Here's the drawing with two shaded views (mm, measured from the low corner). I have some questions. A direction names the side the tool comes from. Coordinates: 2 decimals unless noted, no trailing zeros. Write each loop counter-clockwise with the first axis right and the second up, starting at its lowest first coordinate (ties: lowest second). Pieces come first, ordered by that corner, then holes. Notation, with made-up numbers: (7.5, -34.5) -> (26.5, -34.5) arc R14 ccw to (26.5, -16.5) -> close; hole circle Ø8 at (81, 62.25). An arc over 180 degrees is marked (long way). Answer in a Markdown table with one row per item. Add a question column.
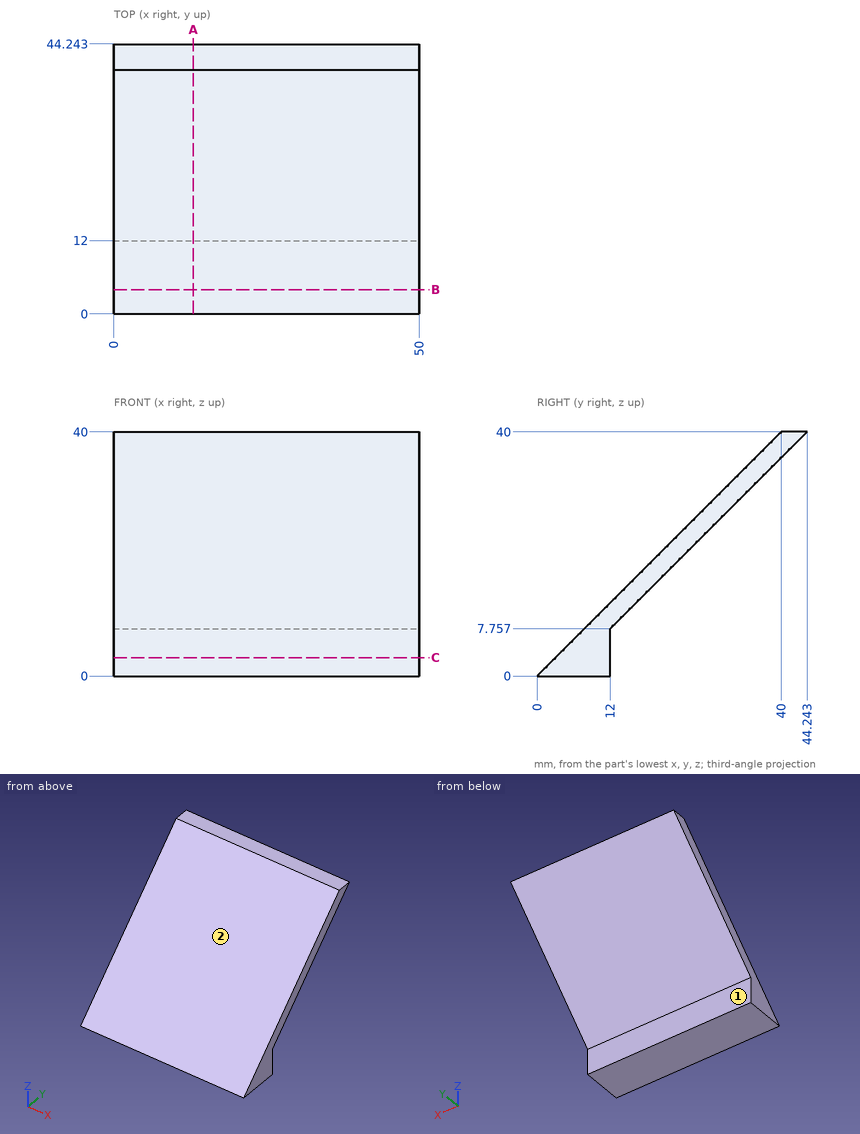
Q1. Imagine slicing it at C-C on z = 3. Please give me the cut outline in (x, y), plus the area to 3 significant figures.
Q2. Imagine slicing it at A-A on x = 13. Please give me the cut outline in (y, z).
Q3. I'm going to push flat-ended pins straight in: P1, Ø6, axis at x = 29.5, z = 5, coming from the +Y side; P2, Ø5, axis at x = 43, z = 26.5, coming from the +Y side; P3, Ø6, axis at x = 14, y = 24, coming from the +Z side. Where does each tip first touch, or does it pass through?
Q4. I need wall thicknesses on line 1 (Y direction, x = 38, z = 24); line 2 (Z direction, x = 17, y = 26.5); line 3 (Y direction, x = 40.5, z = 35). Which ranges of each line are inside material? Lowest first, please. Write a range as [from, to].
Q5. Imagine slicing it at B-B on y = 4. Please give me the cut outline in (x, z).
Q6. For the marked faces 1 and 2, which set-ups out of +Z, -Z, +X, -X, +Y, -Y let a thin tool reach every point of the face, with its end or its side?
Result sheet:
| question | item | result |
|---|---|---|
| 1 | outline | (0, 3) -> (50, 3) -> (50, 12) -> (0, 12) -> close |
| 1 | area | 450 mm^2 |
| 2 | outline | (0, 0) -> (12, 0) -> (12, 7.76) -> (44.24, 40) -> (40, 40) -> close |
| 3 | P1 | stops at y = 12.24 |
| 3 | P2 | stops at y = 33.24 |
| 3 | P3 | stops at z = 27 |
| 4 | line 1 | y = [24, 28.24] |
| 4 | line 2 | z = [22.26, 26.5] |
| 4 | line 3 | y = [35, 39.24] |
| 5 | outline | (0, 0) -> (50, 0) -> (50, 4) -> (0, 4) -> close |
| 6 | face 1 | -Z, +X, -X, +Y |
| 6 | face 2 | +Z, +X, -X, -Y |
